For this review, take the finished solid that the model builds, in its own axes (mm). Coordinates: 2 decimals unless noted, no trailing zeros. Order: outer loops, then holes, each group sorted by start corner. A loop starts at its lowest first (then second) coordinate and runs counter-clockwise, first axis right, second up.
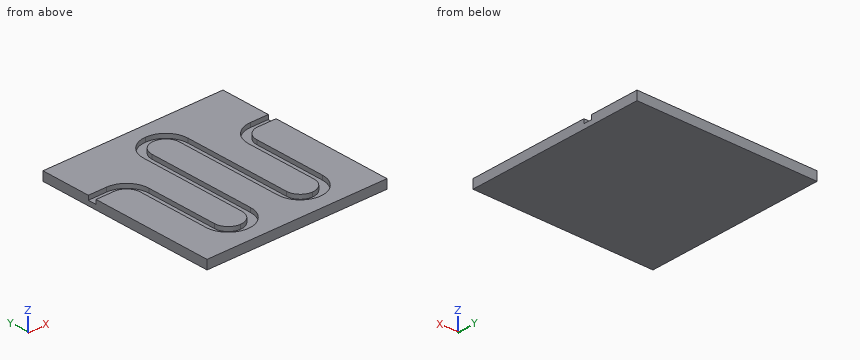
from build123d import *

# Parameters (mm, degrees)
F0_W     = 127
F0_H     = 6.35
F1_DEPTH = 127
F3_W     = 6
F3_H     = 3


with BuildPart() as f1:
    # F0 (on Front) → F1 (new body)
    with BuildSketch(Plane.XZ):
        with Locations((63.5, 3.175)):
            Rectangle(F0_W, F0_H)
    extrude(amount=-F1_DEPTH)

    # F4: sweep along a path in F2
    with BuildLine(Plane.XY.offset(6.35)) as f4_path:
        Line((0, 88.9), (12.7, 88.9))
        ThreePointArc((12.7, 88.9), (21.6802561211, 85.1802561211), (25.4, 76.2))
        Line((25.4, 76.2), (25.4, 25.4))
        ThreePointArc((25.4, 25.4), (29.1197438789, 16.4197438789), (38.1, 12.7))
        ThreePointArc((38.1, 12.7), (47.0802561211, 16.4197438789), (50.8, 25.4))
        Line((50.8, 25.4), (50.8, 76.2))
        Line((50.8, 76.2), (50.8, 101.6))
        ThreePointArc((50.8, 101.6), (54.5197438789, 110.5802561211), (63.5, 114.3))
        ThreePointArc((63.5, 114.3), (72.4802561211, 110.5802561211), (76.2, 101.6))
        Line((76.2, 101.6), (76.2, 76.2))
        Line((76.2, 76.2), (76.2, 25.4))
        ThreePointArc((76.2, 25.4), (79.9197438789, 16.4197438789), (88.9, 12.7))
        ThreePointArc((88.9, 12.7), (97.8802561211, 16.4197438789), (101.6, 25.4))
        Line((101.6, 25.4), (101.6, 76.2))
        ThreePointArc((101.6, 76.2), (105.3197438789, 85.1802561211), (114.3, 88.9))
        Line((114.3, 88.9), (127, 88.9))
    # F3 (on face) → F4 (sweep, cut)
    with BuildSketch(Plane(origin=(0, 0, 0), x_dir=(0, -1, 0), z_dir=(-1, 0, 0))):
        with Locations((-88.9047980309, 4.85)):
            Rectangle(F3_W, F3_H)
    sweep(path=f4_path.line, mode=Mode.SUBTRACT)


solid = f1.part
1. Take a section at A-A, the plane z = 4.75. Give the boundary of the cut face in (x, y).
Answer below:
outline: (0, 0) - (127, 0) - (127, 85.9) - (114.3, 85.9) arc R9.7 ccw to (104.6, 76.2) - (104.6, 25.4) arc R15.7 cw to (73.2, 25.4) - (73.2, 101.6) arc R9.7 ccw to (53.8, 101.6) - (53.8, 25.4) arc R15.7 cw to (22.4, 25.4) - (22.4, 76.2) arc R9.7 ccw to (12.7, 85.9) - (0, 85.9) - close; (0, 91.9) - (12.7, 91.9) arc R15.7 cw to (28.4, 76.2) - (28.4, 25.4) arc R9.7 ccw to (47.8, 25.4) - (47.8, 101.6) arc R15.7 cw to (79.2, 101.6) - (79.2, 25.4) arc R9.7 ccw to (98.6, 25.4) - (98.6, 76.2) arc R15.7 cw to (114.3, 91.9) - (127, 91.9) - (127, 127) - (0, 127) - close
2. Take a section at B-B, the plane y = 100. Give the boundary of the cut face in (x, z).
Answer below:
outline: (0, 0) - (127, 0) - (127, 6.35) - (79.2, 6.35) - (79.2, 3.35) - (73.2, 3.35) - (73.2, 6.35) - (53.8, 6.35) - (53.8, 3.35) - (47.8, 3.35) - (47.8, 6.35) - (0, 6.35) - close
3. Take a section at D-D, the plane y = 31.5. Give the boundary of the cut face in (x, z).
Answer below:
outline: (0, 0) - (127, 0) - (127, 6.35) - (104.6, 6.35) - (104.6, 3.35) - (98.6, 3.35) - (98.6, 6.35) - (79.2, 6.35) - (79.2, 3.35) - (73.2, 3.35) - (73.2, 6.35) - (53.8, 6.35) - (53.8, 3.35) - (47.8, 3.35) - (47.8, 6.35) - (28.4, 6.35) - (28.4, 3.35) - (22.4, 3.35) - (22.4, 6.35) - (0, 6.35) - close
4. To check wall thickness, follow L1, parallel to X at y = 97, z = 3.75; L2, parallel to X at y = 31, z = 4.75; L3, parallel to Y at x = 120.5, z = 3.5. State the ranges of each line that lie inside material, in increasing order.
Answer below:
L1: x = 0 to 47.8, 53.8 to 73.2, 79.2 to 127
L2: x = 0 to 22.4, 28.4 to 47.8, 53.8 to 73.2, 79.2 to 98.6, 104.6 to 127
L3: y = 0 to 85.9, 91.9 to 127
5. Clearance check with flat-ended pins moving along their axes: pin 1 Ø2.5 at (y, z) = (46.5, 5.5) entering from -X; pin 2 Ø2 at (x, y) = (24.5, 36) entering from +Z. State where each tip first meets the part, or that it passes through.
Answer below:
pin 1: stops at x = 0
pin 2: stops at z = 3.35
6. Take a section at C-C, the plane x = 10. Give the boundary of the cut face in (y, z), plus the area to 3 significant figures.
Answer below:
outline: (0, 0) - (127, 0) - (127, 6.35) - (91.9, 6.35) - (91.9, 3.35) - (85.9, 3.35) - (85.9, 6.35) - (0, 6.35) - close
area: 788 mm2
